Input: part model. Units: mm. Frame: model coordinates. Give positions to 0.01 mm unless a question says otherwise; leave off trailing zeros. Loops run counter-clockwise (first coordinate to the right, second up) from the corner with the lowest first, then second, coordinate; pieces in that order, holes last. Notation, with made-up numbers: M -13,61.25 L 32,61.25 A30 ccw 32,96.25 Z; hole C 20,51 d2. An arc over 180 degrees is marked long. Use a Markdown table: item, result. Add a question column.
from build123d import *

# Parameters (mm, degrees)
ESQUISSE1_W                    = 94.6
ESQUISSE1_H                    = 28
BOSS_EXTRU_1_DEPTH             = 3.3
ESQUISSE2_W                    = 8
ESQUISSE2_H                    = 3.3
BOSS_EXTRU_2_DEPTH             = 3.3
R_P_TITION_LIN_AIRE1_COUNT     = 3
R_P_TITION_LIN_AIRE1_PITCH     = 16
R_P_TITION_LIN_AIRE1_COL_COUNT = 4
R_P_TITION_LIN_AIRE1_COL_PITCH = 16
SYM_TRIE1_COPY_1_SKETCH_W      = 8
SYM_TRIE1_COPY_1_SKETCH_H      = 3.3
SYM_TRIE1_COPY_1_DEPTH         = 3.3
SYM_TRIE1_COPY_2_SKETCH_W      = 8
SYM_TRIE1_COPY_2_SKETCH_H      = 3.3
SYM_TRIE1_COPY_2_DEPTH         = 3.3
SYM_TRIE1_COPY_3_SKETCH_W      = 8
SYM_TRIE1_COPY_3_SKETCH_H      = 3.3
SYM_TRIE1_COPY_3_DEPTH         = 3.3
SYM_TRIE1_COPY_4_SKETCH_W      = 8
SYM_TRIE1_COPY_4_SKETCH_H      = 3.3
SYM_TRIE1_COPY_4_DEPTH         = 3.3
SYM_TRIE1_COPY_5_SKETCH_W      = 8
SYM_TRIE1_COPY_5_SKETCH_H      = 3.3
SYM_TRIE1_COPY_5_DEPTH         = 3.3
ESQUISSE3_W                    = 3.3
ESQUISSE3_H                    = 8
ESQUISSE3_H_2                  = 2
ENL_V_MAT_EXTRU_1_DEPTH        = 3.3


with BuildPart() as part:
    # Esquisse1 → Boss.-Extru.1 (new body)
    with BuildSketch(Plane.XY):
        Rectangle(ESQUISSE1_W, ESQUISSE1_H)
    extrude(amount=BOSS_EXTRU_1_DEPTH)

    # Esquisse2 → Boss.-Extru.2 (add)
    with BuildSketch(Plane(origin=(0, 0, 0), x_dir=(-1, 0, 0), z_dir=(0, 0, -1))):
        with Locations((8, 15.65)):
            Rectangle(ESQUISSE2_W, ESQUISSE2_H)
    boss_extru_2 = extrude(amount=-BOSS_EXTRU_2_DEPTH)

    # Répétition linéaire1: Boss.-Extru.2 ×3
    with Locations(*[(-i * R_P_TITION_LIN_AIRE1_PITCH, 0, 0) for i in range(1, R_P_TITION_LIN_AIRE1_COUNT)]):
        add(boss_extru_2)

    # Répétition linéaire1 col: Boss.-Extru.2 ×4
    with Locations(*[(i * R_P_TITION_LIN_AIRE1_COL_PITCH, 0, 0) for i in range(1, R_P_TITION_LIN_AIRE1_COL_COUNT)]):
        add(boss_extru_2)

    # Symétrie1: Boss.-Extru.2 across plane
    add(boss_extru_2.mirror(Plane.ZX))

    # Symétrie1 copy 1 sketch → Symétrie1 copy 1 (add)
    with BuildSketch(Plane(origin=(-16, 0, 0), x_dir=(-1, 0, 0), z_dir=(0, 0, -1))):
        with Locations((8, -15.65)):
            Rectangle(SYM_TRIE1_COPY_1_SKETCH_W, SYM_TRIE1_COPY_1_SKETCH_H)
    extrude(amount=-SYM_TRIE1_COPY_1_DEPTH)

    # Symétrie1 copy 2 sketch → Symétrie1 copy 2 (add)
    with BuildSketch(Plane(origin=(-32, 0, 0), x_dir=(-1, 0, 0), z_dir=(0, 0, -1))):
        with Locations((8, -15.65)):
            Rectangle(SYM_TRIE1_COPY_2_SKETCH_W, SYM_TRIE1_COPY_2_SKETCH_H)
    extrude(amount=-SYM_TRIE1_COPY_2_DEPTH)

    # Symétrie1 copy 3 sketch → Symétrie1 copy 3 (add)
    with BuildSketch(Plane(origin=(16, 0, 0), x_dir=(-1, 0, 0), z_dir=(0, 0, -1))):
        with Locations((8, -15.65)):
            Rectangle(SYM_TRIE1_COPY_3_SKETCH_W, SYM_TRIE1_COPY_3_SKETCH_H)
    extrude(amount=-SYM_TRIE1_COPY_3_DEPTH)

    # Symétrie1 copy 4 sketch → Symétrie1 copy 4 (add)
    with BuildSketch(Plane(origin=(32, 0, 0), x_dir=(-1, 0, 0), z_dir=(0, 0, -1))):
        with Locations((8, -15.65)):
            Rectangle(SYM_TRIE1_COPY_4_SKETCH_W, SYM_TRIE1_COPY_4_SKETCH_H)
    extrude(amount=-SYM_TRIE1_COPY_4_DEPTH)

    # Symétrie1 copy 5 sketch → Symétrie1 copy 5 (add)
    with BuildSketch(Plane(origin=(48, 0, 0), x_dir=(-1, 0, 0), z_dir=(0, 0, -1))):
        with Locations((8, -15.65)):
            Rectangle(SYM_TRIE1_COPY_5_SKETCH_W, SYM_TRIE1_COPY_5_SKETCH_H)
    extrude(amount=-SYM_TRIE1_COPY_5_DEPTH)

    # Esquisse3 → Enlèv. mat.-Extru.1 (cut)
    with BuildSketch(Plane(origin=(0, 0, 0), x_dir=(-1, 0, 0), z_dir=(0, 0, -1))):
        with Locations((-45.65, 0)):
            Rectangle(ESQUISSE3_W, ESQUISSE3_H)
        with Locations((-45.65, 13)):
            Rectangle(ESQUISSE3_W, ESQUISSE3_H_2)
        with Locations((-45.65, -13)):
            Rectangle(ESQUISSE3_W, ESQUISSE3_H_2)
    enl_v_mat_extru_1 = extrude(amount=-ENL_V_MAT_EXTRU_1_DEPTH, mode=Mode.SUBTRACT)

    # Symétrie2: Enlèv. mat.-Extru.1 across plane
    add(enl_v_mat_extru_1.mirror(Plane(origin=(0, 0, 0), x_dir=(0, 0, 1), z_dir=(1, 0, 0))), mode=Mode.SUBTRACT)


solid = part.part
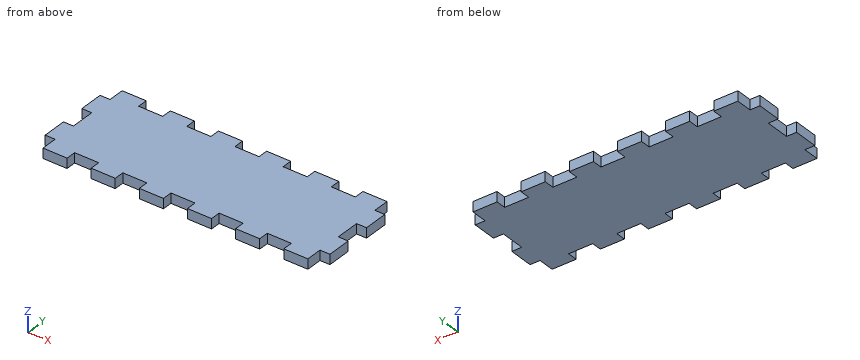
1) Section query A-A, the plane y = -0.5. Return the cut outline in (x, z), and give its area (3 significant figures).
2) Contact query for flat-ended pins moving along their axis: P1, Ø1.6, axis at y = 15.5, z = 2, coming from the -X side; P2, Ø1, axis at y = 15.5, z = 1.5, coming from the +X side; P3, Ø1, axis at x = -35, z = 0.5, coming from the -Y side. Output: stop coordinate, or through.
3) Ray query, line 1 (X direction, y = 15, z = 1.4); line 2 (Y direction, x = 17, z = 0.3); line 3 (X direction, y = 1, z = 1.05). Return the intervals inside material, ascending. Write a range as [from, to].
4) Section query B-B, the plane x = -14. Return the cut outline in (y, z).
Entries:
| question | item | result |
|---|---|---|
| 1 | outline | M -44,0 L 44,0 L 44,3.3 L -44,3.3 Z |
| 1 | area | 290 mm² |
| 2 | P1 | stops at x = -44 |
| 2 | P2 | stops at x = 44 |
| 2 | P3 | stops at y = -14 |
| 3 | line 1 | x = [-44, -36], [-28, -20], [-12, -4], [4, 12], [20, 28], [36, 44] |
| 3 | line 2 | y = [-14, 14] |
| 3 | line 3 | x = [-44, 44] |
| 4 | outline | M -14,0 L 14,0 L 14,3.3 L -14,3.3 Z |
